from build123d import *

# Parameters (mm, degrees)
F0_R     = 14.2875
F1_DEPTH = 2.54
F2_R     = 14.2875
F2_R_2   = 13.0175
F3_DEPTH = 6.35
F4_DEPTH = 6.35
F5_R     = 2.54
F6_DEPTH = 25.4


with BuildPart() as f1:
    # F0 (on Top) → F1 (new body)
    with BuildSketch(Plane.XY):
        Circle(F0_R)
    extrude(amount=F1_DEPTH)

    # F2 (on face) → F3 (join)
    with BuildSketch(Plane(origin=(0, 0, 0), x_dir=(1, 0, 0), z_dir=(0, 0, -1))):
        Circle(F2_R)
        Circle(F2_R_2, mode=Mode.SUBTRACT)
    extrude(amount=F3_DEPTH)

    # F2 (on face) → F4 (join, through all)
    with BuildSketch(Plane(origin=(0, 0, 0), x_dir=(1, 0, 0), z_dir=(0, 0, -1))):
        with BuildLine():
            Line((0, 10.7315), (0, 11.7475))
            ThreePointArc((0, 11.7475), (-5.87375, 10.173633), (-10.173633, 5.87375))
            Line((-10.173633, 5.87375), (-9.293752, 5.36575))
            ThreePointArc((-9.293752, 5.36575), (-5.36575, 9.293752), (0, 10.7315))
        make_face()
    extrude(amount=F4_DEPTH)

    # F5 (on face) → F6 (cut)
    with BuildSketch(Plane(origin=(0, 0, 0), x_dir=(1, 0, 0), z_dir=(0, 0, -1))):
        Circle(F5_R)
    extrude(amount=-F6_DEPTH, mode=Mode.SUBTRACT)


solid = f1.part
Geometry: final body of the model. Coordinates: model frame, mm. A direction names the side the tool comes from. Give positions to 0.01 mm unless a question says otherwise; leave off trailing zeros. Loops run counter-clockwise (first coordinate to the right, second up) from the corner with the lowest first, then second, coordinate; pieces in that order, holes last. Notation, with made-up numbers: (-12.5, -17) -> (12.5, -17) arc R23 ccw to (12.5, 17) -> close; hole circle Ø6 at (32.5, 2.25). An arc over 180 degrees is marked (long way). Put each result on its own line as item: value.
1. Set-up query: faces 1 (the cylindrical face through (-0.33, -2.52, 1.25)), 2 (the flat face through (-9.7, -5.6, -3.1)). Return all of +Z, -Z, +X, -X, +Y, -Y with unobstructed straight access to the full face (end or side cutting, diameter ignored); none if empty.
Taken from the geometry:
face 1: +Z, -Z
face 2: -Z
2. Ray query, line 1 along X through (y, z) = (0, -1.25); line 2 along Y through (x, z) = (-3.5, -2); line 3 along Y through (x, z) = (-7, -5.5). Return the intervals inside material, ascending. Write a range as [from, to].
Taken from the geometry:
line 1: x = [-14.29, -13.02], [13.02, 14.29]
line 2: y = [-13.85, -12.54], [-11.21, -10.14], [12.54, 13.85]
line 3: y = [-12.46, -10.98], [-9.43, -8.13], [10.98, 12.46]
3. Cut plane D-D (y = -3). Return the cut outline in (x, z), plus the area to 3 significant figures.
Taken from the geometry:
outline: (-13.97, -6.35) -> (-12.67, -6.35) -> (-12.67, 0) -> (12.67, 0) -> (12.67, -6.35) -> (13.97, -6.35) -> (13.97, 2.54) -> (-13.97, 2.54) -> close
area: 87.5 mm2
4. Pin query (flat end, axial travel): P1, Ø2, axis at x = -2, z = -1.5, coming from the -Y side; P2, Ø4, axis at y = 9.5, z = -1, coming from the +X side; P3, Ø3, axis at x = 6, z = -1, coming from the +Y side. Return the tip coordinate at first contact, or that it passes through.
Taken from the geometry:
P1: stops at y = -14.25
P2: stops at x = 12.16
P3: stops at y = 13.56
5. Cut plane C-C (x = 8.75). Return the cut outline in (y, z), plus the area to 3 significant figures.
Taken from the geometry:
outline: (-11.29, -6.35) -> (-9.64, -6.35) -> (-9.64, 0) -> (9.64, 0) -> (9.64, -6.35) -> (11.29, -6.35) -> (11.29, 2.54) -> (-11.29, 2.54) -> close
area: 78.4 mm2
6. Cut plane A-A (z = -4.75). Return the cut outline in (x, y) (1 decimal).
Taken from the geometry:
outline: circle Ø28.6 at (0, 0); (-10.2, -5.9) arc R11.7 ccw to (0, -11.7) -> (0, -10.7) arc R10.7 cw to (-9.3, -5.4) -> close; hole circle Ø26 at (0, 0)
7. Pull-direction query (X, two-part tool) for faces 3 (the flat face through (3, 0, 0)), 4 (the cylindrical face through (-14.274, -0.628, -1.843)), 5 (the flat face through (-5, -10, -6.35)); classes: released by +X, released by -X, zero draft, split by the parting line, or undercut.
Taken from the geometry:
face 3: undercut
face 4: split by the parting line
face 5: zero draft
8. Cut plane B-B (y = 0). Return the cut outline in (x, z), plus the area to 3 significant figures.
Taken from the geometry:
outline: (-14.29, -6.35) -> (-13.02, -6.35) -> (-13.02, 0) -> (-2.54, 0) -> (-2.54, 2.54) -> (-14.29, 2.54) -> close; (2.54, 0) -> (13.02, 0) -> (13.02, -6.35) -> (14.29, -6.35) -> (14.29, 2.54) -> (2.54, 2.54) -> close
area: 75.8 mm2
